from build123d import *

# Parameters (mm, degrees)
SKETCH1_R             = 52.3875
SKETCH1_R_2           = 23.5
BOSS_EXTRUDE1_DEPTH   = 5.715
M6_CLEARANCE_HOLE1_D  = 6.6
F_5_0MM_DOWEL_HOLE1_D = 5
CIRPATTERN1_COUNT     = 4
CUT_EXTRUDE1_DEPTH    = 284.979078357
CUT_EXTRUDE2_DEPTH    = 284.979078357


with BuildPart() as part:
    # Sketch1 → Boss-Extrude1 (new, symmetric)
    with BuildSketch(Plane(origin=(0, 0, 0), x_dir=(1, 0, 0), z_dir=(0, 1, 0))):
        with BuildLine():
            Line((-207.974881785, -9.956762437), (-62.780706514, -68.14502812))
            ThreePointArc((-62.780706514, -68.14502812), (-33.518744337, -68.231765471), (-12.176603989, -48.212200061))
            Line((-12.176603989, -48.212200061), (1.412558245, -19.284326264))
            ThreePointArc((1.412558245, -19.284326264), (9.247910088, -13.841666007), (17.871565555, -17.92184438))
            Line((17.871565555, -17.92184438), (44.159519082, -55.990558325))
            ThreePointArc((44.159519082, -55.990558325), (54.61, -61.474087679), (65.060480918, -55.990558325))
            Line((65.060480918, -55.990558325), (91.348434445, -17.92184438))
            ThreePointArc((91.348434445, -17.92184438), (102.948934458, -14.583873353), (108.5062916, -25.299722957))
            Line((108.5062916, -25.299722957), (85.67665489, -133.551751975))
            ThreePointArc((85.67665489, -133.551751975), (75.916532775, -150.539204768), (58.043657912, -158.563784522))
            Line((58.043657912, -158.563784522), (-116.494367072, -177.55085719))
            ThreePointArc((-116.494367072, -177.55085719), (-142.092740129, -174.957766874), (-164.426538493, -162.182702446))
            ThreePointArc((-164.426538493, -162.182702446), (-168.164823601, -160.06920649), (-172.443362527, -159.700770109))
            Line((-172.443362527, -159.700770109), (-204.355245166, -163.82191268))
            ThreePointArc((-204.355245166, -163.82191268), (-214.295764489, -158.206433226), (-211.707233022, -147.086764223))
            Line((-211.707233022, -147.086764223), (-198.151371623, -135.681934472))
            ThreePointArc((-198.151371623, -135.681934472), (-188.283833694, -119.954004575), (-189.430137427, -101.422354045))
            Line((-189.430137427, -101.422354045), (-220.388836369, -22.267635732))
            ThreePointArc((-220.388836369, -22.267635732), (-218.225236723, -12.034965467), (-207.974881785, -9.956762437))
        make_face()
        with Locations(Location((-123.19, -116.001477372, 0), (0, 0, 270))):
            Circle(SKETCH1_R, mode=Mode.SUBTRACT)
        with Locations(Location((54.61, -127, 0), (0, 0, 270))):
            Circle(SKETCH1_R_2, mode=Mode.SUBTRACT)
    extrude(amount=BOSS_EXTRUDE1_DEPTH, both=True)

    # M6 Clearance Hole1 (through all)
    with Locations(Plane(origin=(0, -5.715, 0), x_dir=(-1, 0, 0), z_dir=(0, -1, 0))):
        with Locations((-10.033704867, -23.334197365), (211.518182886, -18.798178744), (205.575185514, -154.375359311), (-99.186295133, -23.334197365)):
            Hole(M6_CLEARANCE_HOLE1_D / 2)

    # Ø5.0mm Dowel Hole1 (through all)
    with Locations(Plane(origin=(0, -5.715, 0), x_dir=(-1, 0, 0), z_dir=(0, -1, 0))):
        with Locations((123.19, -173.151477372)):
            f_5_0mm_dowel_hole1 = Hole(F_5_0MM_DOWEL_HOLE1_D / 2)

    # CirPattern1: Ø5.0mm Dowel Hole1 ×4 about axis
    cirpattern1_axis = Axis((-123.19, 0, 116.001477372), (0, 1, 0))
    for i in range(1, CIRPATTERN1_COUNT):
        add(f_5_0mm_dowel_hole1.rotate(cirpattern1_axis, i * 360 / CIRPATTERN1_COUNT), mode=Mode.SUBTRACT)

    # Sketch6 → Cut-Extrude1 (cut, through all)
    with BuildSketch(Plane.XZ.offset(5.715)):
        with BuildLine():
            ThreePointArc((-14.234653979, 76.580666612), (-13.797169823, 82.649279585), (-8.456504121, 85.564197365))
            Line((-8.456504121, 85.564197365), (41.801580719, 85.564197365))
            ThreePointArc((41.801580719, 85.564197365), (47.441443369, 82.132150292), (46.984841737, 75.545913676))
            Line((46.984841737, 75.545913676), (21.201297863, 39.113933708))
            ThreePointArc((21.201297863, 39.113933708), (11.084872861, 34.469497273), (2.016277078, 40.924992231))
            Line((2.016277078, 40.924992231), (-14.234653979, 76.580666612))
        make_face()
        with BuildLine():
            ThreePointArc((-188.626913597, 77.326218823), (-183.343464985, 81.400582198), (-177.265672517, 78.648182362))
            ThreePointArc((-177.265672517, 78.648182362), (-164.864290964, 65.181201114), (-149.229324423, 55.657458697))
            ThreePointArc((-149.229324423, 55.657458697), (-145.319075006, 49.625624375), (-149.386073966, 43.698348841))
            Line((-149.386073966, 43.698348841), (-194.042740287, 25.801666969))
            ThreePointArc((-194.042740287, 25.801666969), (-202.810079512, 27.579196728), (-204.660650751, 36.331409888))
            Line((-204.660650751, 36.331409888), (-188.626913597, 77.326218823))
        make_face()
        with BuildLine():
            ThreePointArc((-194.692687992, 140.689511725), (-195.773357295, 149.809803058), (-188.096484537, 154.850952212))
            Line((-188.096484537, 154.850952212), (-182.142551509, 155.01295786))
            ThreePointArc((-182.142551509, 155.01295786), (-179.298484939, 153.425933155), (-179.332786017, 150.169219243))
            ThreePointArc((-179.332786017, 150.169219243), (-182.766707481, 143.751485155), (-185.46990532, 136.993390091))
            ThreePointArc((-185.46990532, 136.993390091), (-187.940827525, 134.871620657), (-190.985681304, 136.027573744))
            Line((-190.985681304, 136.027573744), (-194.692687992, 140.689511725))
        make_face()
    extrude(amount=-CUT_EXTRUDE1_DEPTH, mode=Mode.SUBTRACT)

    # Sketch7 → Cut-Extrude2 (cut, through all)
    with BuildSketch(Plane.XZ.offset(5.715)):
        with BuildLine():
            Line((-48.815667356, 114.096477372), (7.572332644, 114.096477372))
            ThreePointArc((7.572332644, 114.096477372), (17.097332644, 104.571477372), (7.572332644, 95.046477372))
            Line((7.572332644, 95.046477372), (-48.815667356, 95.046477372))
            ThreePointArc((-48.815667356, 95.046477372), (-58.340667356, 104.571477372), (-48.815667356, 114.096477372))
        make_face()
        with BuildLine():
            Line((-60.480063265, 159.980626251), (9.143311078, 148.338049571))
            ThreePointArc((9.143311078, 148.338049571), (17.064665217, 138.155302762), (7.572332644, 129.418495204))
            Line((7.572332644, 129.418495204), (-51.525154545, 129.418495204))
            ThreePointArc((-51.525154545, 129.418495204), (-57.140513894, 131.249772802), (-60.59665397, 136.039442314))
            ThreePointArc((-60.59665397, 136.039442314), (-63.415414116, 143.322639291), (-67.078188304, 150.220062883))
            ThreePointArc((-67.078188304, 150.220062883), (-66.914295931, 157.219714512), (-60.480063265, 159.980626251))
        make_face()
    extrude(amount=-CUT_EXTRUDE2_DEPTH, mode=Mode.SUBTRACT)


solid = part.part
Verification items for the finished model (mm, model axes). A direction names the side the tool comes from. Coordinates: 2 decimals unless noted, no trailing zeros. Order: outer loops, then holes, each group sorted by start corner. A loop starts at its lowest first (then second) coordinate and runs counter-clockwise, first axis right, second up. Notation, with made-up numbers: M 82,0.5 L 138,0.5 A24 cw 138,10.5 Z; hole C 76,-17.75 d8. An arc over 180 degrees is marked long. Write each question's results on one line, items separated by ' | '.
1) Gauge pin test, flat ends, axial feed: pin 1 Ø6 at (y, z) = (0, 104) entering from +X; pin 2 Ø1 at (x, y) = (-153, 2) entering from +Z; pin 3 Ø1.5 at (y, z) = (2.5, 150.5) entering from +X; pin 4 Ø6 at (x, z) = (-123.19, 58.85) entering from -Y (3 decimals). Record the tip position at first contact, or that the pin passes through.
Solved:
pin 1: stops at x = 92.54 | pin 2: stops at z = 170.54 | pin 3: stops at x = 76.76 | pin 4: stops at y = -5.715
2) Section check B-B on x = -42. Record the cut outline in (y, z) (1 decimal), plus the area to 3 significant figures.
Solved:
outline: M -5.7,70.5 L 5.7,70.5 L 5.7,95 L -5.7,95 Z; M -5.7,114.1 L 5.7,114.1 L 5.7,129.4 L -5.7,129.4 Z; M -5.7,156.9 L 5.7,156.9 L 5.7,169.4 L -5.7,169.4 Z | area: 599 mm²
3) Section check A-A on x = -107.5. Record the cut outline in (y, z) (3 decimals), plus the area to 3 significant figures.
Solved:
outline: M -5.715,50.223 L 5.715,50.223 L 5.715,66.019 L -5.715,66.019 Z; M -5.715,165.984 L 5.715,165.984 L 5.715,176.572 L -5.715,176.572 Z | area: 302 mm²
4) Section check C-C on x = 75. Record the cut outline in (y, z) (3 decimals).
Solved:
outline: M -5.715,41.597 L 5.715,41.597 L 5.715,115.317 L -5.715,115.317 Z; M -5.715,138.683 L 5.715,138.683 L 5.715,151.337 L -5.715,151.337 Z
5) Scan lines: line 1 along Z through (x, y) = (-165.5, -2.75); line 2 along Z through (x, y) = (-33.5, -3.25); line 3 along X through (y, z) = (0, 59). Record each from-to range of solid material in increasing order. Write a range as [from, to].
Solved:
line 1: z = [26.98, 37.24], [65.71, 85.11], [146.89, 161.35] | line 2: z = [68.22, 95.05], [114.1, 129.42], [155.47, 168.52] | line 3: x = [-206.02, -195.79], [-155.91, -125.69], [-120.69, -85.6], [-19.64, -6.22], [35.28, 47.08], [62.14, 101.4]
6) Access from +Z, -Z, +X, -X, +Y, -Y to the whole of each face (thin tool, end or side, straight path). Record for faces 1 (the face through (-136.394, 0.08, 38.644)), 2 (the face through (-204.693, 0.08, 62.399)), 3 (the face through (-168.107, 0.08, 160.087)), 4 (the face through (-43, -5.715, 81)), 5 (the face through (17.095, -0.08, 104.781)).
Solved:
face 1: -Z, +Y, -Y | face 2: -X, +Y, -Y | face 3: +Z, +Y, -Y | face 4: +Z, -Z, +X, -X, -Y | face 5: +Y, -Y
7) Release check for a two-part mould opening along Z. For faces 6 (the face through (-205.02, 0.08, 141.46)), 7 (the face through (-33.91, 0.08, 68.383)), 8 (the face through (-141.747, 0.08, 175.068)) record: pulls with the +Z half, pulls with the -Z half, needs draft (parallel to the pull), parting line crosses it, or undercut.
Solved:
face 6: undercut | face 7: pulls with the -Z half | face 8: pulls with the +Z half
8) Section check D-D on y = -1.5. Give the number of separate pieces and of enclosed holes in the cut face, plus the area to 3 significant figures.
Solved:
separate pieces: 1 | enclosed holes: 15 | area: 18,800 mm²
